from build123d import *

# Parameters (mm, degrees)
LINEAR_AUSTRAGEN_D_NN1_OUTLINE_R = 35
LINEAR_AUSTRAGEN_D_NN1_DEPTH     = 3
F_5_7_5_7_DURCHMESSER_BOHRUNG1_D = 5.7
KREISMUSTER1_COUNT               = 21


# Read off the part's stored shape, not the designer's step: Linear-Austragen-Dünn1
with BuildPart() as part:
    # Linear-Austragen-Dünn1 outline → Linear-Austragen-Dünn1 (new body)
    with BuildSketch(Plane(origin=(0, 0, 0), x_dir=(0, 0, -1), z_dir=(1, 0, 0))):
        with BuildLine():
            ThreePointArc((39.8, -3.994996871), (44, 0), (39.8, 3.994996871))
            ThreePointArc((39.8, 3.994996871), (39.553233049, 5.961690647), (39.20934367, 7.913745572))
            ThreePointArc((39.20934367, 7.913745572), (42.045203455, 12.969227674), (36.854251671, 15.548766311))
            ThreePointArc((36.854251671, 15.548766311), (36.038754716, 17.355349565), (35.134765087, 19.119316993))
            ThreePointArc((35.134765087, 19.119316993), (36.35450607, 24.786082555), (30.633841348, 25.720959629))
            ThreePointArc((30.633841348, 25.720959629), (29.322074873, 27.206909511), (27.93830844, 28.626053195))
            ThreePointArc((27.93830844, 28.626053195), (27.433551282, 34.400585229), (21.691479788, 33.60773281))
            ThreePointArc((21.691479788, 33.60773281), (20, 34.641016151), (18.259410483, 35.589238947))
            ThreePointArc((18.259410483, 35.589238947), (16.075005072, 40.95844494), (10.821735057, 38.508311445))
            ThreePointArc((10.821735057, 38.508311445), (8.900837358, 38.997116487), (6.958083774, 39.390164638))
            ThreePointArc((6.958083774, 39.390164638), (3.288124118, 43.876967076), (-1.009568325, 39.987257618))
            ThreePointArc((-1.009568325, 39.987257618), (-2.989203744, 39.888151887), (-4.961499213, 39.69110134))
            ThreePointArc((-4.961499213, 39.69110134), (-9.790921094, 42.896828136), (-12.75116713, 37.91316047))
            ThreePointArc((-12.75116713, 37.91316047), (-14.613640975, 37.234949946), (-16.440231222, 36.465309506))
            ThreePointArc((-16.440231222, 36.465309506), (-22, 38.105117767), (-23.359768778, 32.470312635))
            ThreePointArc((-23.359768778, 32.470312635), (-24.939592074, 31.273259299), (-26.45817654, 29.999414898))
            ThreePointArc((-26.45817654, 29.999414898), (-32.254282361, 29.927600462), (-31.892752458, 24.142335029))
            ThreePointArc((-31.892752458, 24.142335029), (-33.049550973, 22.532802323), (-34.125196762, 20.867940625))
            ThreePointArc((-34.125196762, 20.867940625), (-39.642630188, 19.090884522), (-37.591925123, 13.669205009))
            ThreePointArc((-37.591925123, 13.669205009), (-38.222912231, 11.790206977), (-38.760043497, 9.882258251))
            ThreePointArc((-38.760043497, 9.882258251), (-43.508556354, 6.557859712), (-39.950890271, 1.981506137))
            ThreePointArc((-39.950890271, 1.981506137), (-40, 0), (-39.950890271, -1.981506137))
            ThreePointArc((-39.950890271, -1.981506137), (-43.508556354, -6.557859712), (-38.760043497, -9.882258251))
            ThreePointArc((-38.760043497, -9.882258251), (-38.222912231, -11.790206977), (-37.591925123, -13.669205009))
            ThreePointArc((-37.591925123, -13.669205009), (-39.642630188, -19.090884522), (-34.125196762, -20.867940625))
            ThreePointArc((-34.125196762, -20.867940625), (-33.049550973, -22.532802323), (-31.892752458, -24.142335029))
            ThreePointArc((-31.892752458, -24.142335029), (-32.254282361, -29.927600462), (-26.45817654, -29.999414898))
            ThreePointArc((-26.45817654, -29.999414898), (-24.939592074, -31.273259299), (-23.359768778, -32.470312635))
            ThreePointArc((-23.359768778, -32.470312635), (-22, -38.105117767), (-16.440231222, -36.465309506))
            ThreePointArc((-16.440231222, -36.465309506), (-14.613640975, -37.234949946), (-12.75116713, -37.91316047))
            ThreePointArc((-12.75116713, -37.91316047), (-9.790921094, -42.896828136), (-4.961499213, -39.69110134))
            ThreePointArc((-4.961499213, -39.69110134), (-2.989203744, -39.888151887), (-1.009568325, -39.987257618))
            ThreePointArc((-1.009568325, -39.987257618), (3.288124118, -43.876967076), (6.958083774, -39.390164638))
            ThreePointArc((6.958083774, -39.390164638), (8.900837358, -38.997116487), (10.821735057, -38.508311445))
            ThreePointArc((10.821735057, -38.508311445), (16.075005072, -40.95844494), (18.259410483, -35.589238947))
            ThreePointArc((18.259410483, -35.589238947), (20, -34.641016151), (21.691479788, -33.60773281))
            ThreePointArc((21.691479788, -33.60773281), (27.433551282, -34.400585229), (27.93830844, -28.626053195))
            ThreePointArc((27.93830844, -28.626053195), (29.322074873, -27.206909511), (30.633841348, -25.720959629))
            ThreePointArc((30.633841348, -25.720959629), (36.35450607, -24.786082555), (35.134765087, -19.119316993))
            ThreePointArc((35.134765087, -19.119316993), (36.038754716, -17.355349565), (36.854251671, -15.548766311))
            ThreePointArc((36.854251671, -15.548766311), (42.045203455, -12.969227674), (39.20934367, -7.913745572))
            ThreePointArc((39.20934367, -7.913745572), (39.553233049, -5.961690647), (39.8, -3.994996871))
        make_face()
        Circle(LINEAR_AUSTRAGEN_D_NN1_OUTLINE_R, mode=Mode.SUBTRACT)
    extrude(amount=LINEAR_AUSTRAGEN_D_NN1_DEPTH)

    # Ø5.7 (5.7) Durchmesser Bohrung1 (through all)
    with Locations(Plane(origin=(3, 0, 0), x_dir=(0, 0, -1), z_dir=(1, 0, 0))):
        with Locations((40, 0)):
            f_5_7_5_7_durchmesser_bohrung1 = Hole(F_5_7_5_7_DURCHMESSER_BOHRUNG1_D / 2)

    # Kreismuster1: Ø5.7 (5.7) Durchmesser Bohrung1 ×21 about axis
    kreismuster1_axis = Axis((0, 0, 0), (1, 0, 0))
    for i in range(1, KREISMUSTER1_COUNT):
        add(f_5_7_5_7_durchmesser_bohrung1.rotate(kreismuster1_axis, i * 360 / KREISMUSTER1_COUNT), mode=Mode.SUBTRACT)


solid = part.part
Read the model definition and answer for the solid it produces. Units are mm, in the model's axes. A direction names the side the tool comes from. Round coordinates to 2 decimals unless told otherwise and drop trailing zeros. Order: outer loops, then holes, each group sorted by start corner. A loop starts at its lowest first (then second) coordinate and runs counter-clockwise, first axis right, second up.
1) For faces 1 (the face through (1.48, 31.29, 24.92)), 2 (the face through (0, 20, 29)), determine the directions among +Z, -Z, +X, -X, +Y, -Y from which every point of the face is accessible in a straight line to the end or side of a thin tool.
2) Flat-ended cylindrical pins translate along their axes: pin 1 (5 mm diameter, centred on y = -17.36, z = 36.04, fed in from +X); pin 2 (1.5 mm diameter, centred on x = 1, y = 27, fed in from +Z). Find the tip coordinate at first contact, or state that the pin passes through.
3) The mould has two halves that part along Z. Classify faces 3 (the face through (1.48, -16.77, 38.83)), 4 (the face through (1.479, -1.092, -37.367)), 5 (the face through (3, 20, 29)): released by +Z, released by -Z, zero draft, split by the parting line, or undercut.
4) The part is cut by section C-C on x = 0.6. Give the number of separate pieces and of enclosed holes in the cut face, plus the area to 3 significant figures.
5) The part is cut by section A-A on y = 0. Write down the section's boundary in (x, z), plus the area to 3 significant figures.
6) Straight lines are drawn through the part: L1, parallel to Z at x = 1.55, y = 6; L2, parallel to Z at x = 2.65, y = -29; L3, parallel to Y at x = 1.5, z = 6.5. For each, find the intervals that lie inside material, in ascending order.
7) The part is cut by section B-B on z = 20. Write down the section's boundary in (x, y), plus the area to 3 significant figures.
Resolved:
1. face 1: +X, -X
1. face 2: +Z, -Z, -X, +Y, -Y
2. pin 1: passes through
2. pin 2: stops at z = 33.32
3. face 3: undercut
3. face 4: undercut
3. face 5: zero draft
4. separate pieces: 1
4. enclosed holes: 22
4. area: 1,180 mm2
5. outline: (0, -44) - (3, -44) - (3, -42.85) - (0, -42.85) - close; (0, -37.15) - (3, -37.15) - (3, -35) - (0, -35) - close; (0, 35) - (3, 35) - (3, 40) - (0, 40) - close
5. area: 24.9 mm2
6. L1: z = -39.55 to -34.48, 34.48 to 36.7, 42.4 to 43.55
6. L2: z = -28.23 to -26.66, -23.22 to -19.6, 19.6 to 27.11, 31.54 to 32.9
6. L3: y = -42.2 to -40.53, -37.46 to -34.39, 34.39 to 37.46, 40.53 to 42.2
7. outline: (0, -38.64) - (3, -38.64) - (3, -37.49) - (0, -37.49) - close; (0, -31.79) - (3, -31.79) - (3, -28.72) - (0, -28.72) - close; (0, 28.72) - (3, 28.72) - (3, 31.79) - (0, 31.79) - close; (0, 37.49) - (3, 37.49) - (3, 38.64) - (0, 38.64) - close
7. area: 25.3 mm2
